Geometry: final body of the model. Coordinates: model frame, mm. Coordinates: 2 decimals unless noted, no trailing zeros. Order: outer loops, then holes, each group sorted by start corner. A loop starts at its lowest first (then second) coordinate and runs counter-clockwise, first axis right, second up. Notation, with made-up numbers: M 36,-15.5 L 95,-15.5 A12 ccw 95,-8.5 Z; hole C 52.25,67 d1. An arc over 180 degrees is marked long. Write item = value, one per line.
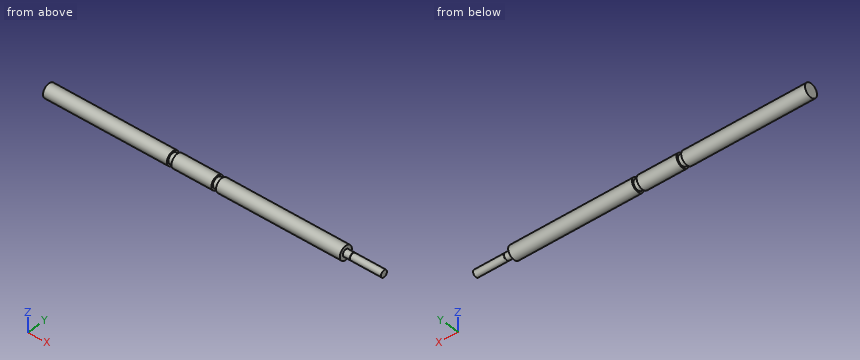
from build123d import *


with BuildPart() as f1:
    # F0 (on Front) → F1 (revolve)
    with BuildSketch(Plane.XZ):
        Polygon((146, 16), (0, 16), (0, 8), (358, 8), (358.9, 8), (395, 8), (395, 12), (358.9, 12), (358.9, 11.8), (358, 11.8), (358, 12), (350, 12), (350, 16), (204, 16), (204, 14), (198.5, 14), (198.5, 16), (151.5, 16), (151.5, 14), (146, 14), align=None)
    revolve(axis=Axis((197.5, 0, 8), (1, 0, 0)))


solid = f1.part
1) Section C-C, the plane x = 256. Return loops of the section in (y, z).
Numbers:
outline = C 0,8 d16
2) Line query: L1, parallel to X at y = 5.75, z = 3.5; L2, parallel to Z at x = 295, y = 7; L3, parallel to X at y = 1, z = 13. Output: solid intervals per line, ascending.
Numbers:
L1 = 0 to 146, 151.5 to 198.5, 204 to 350
L2 = 4.13 to 11.87
L3 = 0 to 350
3) Pin query (flat end, axial travel): pin 1 (8 mm diameter, centred on x = 52, z = 2.5, fed in from +Y); pin 2 (2 mm diameter, centred on x = 120.5, z = 6.5, fed in from -Y). Return the tip coordinate at first contact, or that it passes through.
Numbers:
pin_1 = 7.86
pin_2 = -7.98
